```python
from build123d import *

# Parameters (mm, degrees)
F2_DEPTH = 10


with BuildPart() as f2:
    # F0 (on Front) → F2 (new body)
    with BuildSketch(Plane.XZ):
        with BuildLine():
            Line((0.211261, 25.041597), (0, 26.312215))
            ThreePointArc((0, 26.312215), (-0.220003, 26.826498), (-0.481302, 27.32108))
            ThreePointArc((-0.481302, 27.32108), (-0.825797, 27.312847), (-1.170161, 27.300274))
            ThreePointArc((-1.170161, 27.300274), (-1.401135, 26.790824), (-1.589699, 26.264201))
            Line((-1.589699, 26.264201), (-1.724216, 24.980969))
            Line((-1.724216, 24.980969), (-3.022362, 24.863022))
            Line((-3.022362, 24.863022), (-0.476655, 3.921135))
            ThreePointArc((-0.476655, 3.921135), (-0.222131, 3.943749), (0.033323, 3.949859))
            Line((0.033323, 3.949859), (0.211261, 25.041597))
        make_face()
    extrude(amount=F2_DEPTH)


with BuildPart() as f2_1:
    # F3: moved
    add(f2.part.moved(Location((0, 0, 0.5))))


solid = f2_1.part
```
Check sheet for the modelled part. Datum: model origin and axes. Units: mm. Coordinates: 2 decimals unless noted, no trailing zeros. Order: outer loops, then holes, each group sorted by start corner. A loop starts at its lowest first (then second) coordinate and runs counter-clockwise, first axis right, second up. Notation, with made-up numbers: (67, 25) -> (114, 25) arc R18 ccw to (114, 30) -> close; hole circle Ø2 at (-14.5, 48). An arc over 180 degrees is marked (long way). Write each question's results on one line, items separated by ' | '. Start each with the question number.
1) Draft check along Z on faces 1 (the face through (-1.767, -4.93, 15.039)), 2 (the face through (-1, 0, 19)), 3 (the face through (-1.398, -4.93, 27.298)). Enter one of: pulls with the +Z half, pulls with the -Z half, needs draft (parallel to the pull), parting line crosses it, or undercut.
2) Section check C-C (x = -0.7). Enter the section's corners in (y, z), and give its area (3 significant figures).
3) Section check A-A (y = -1). Enter the section's corners in (x, z), and give its area (3 significant figures).
4) Material ranges on line 1 along X through (y, z) = (-4.5, 18); line 2 along X through (y, z) = (-0.25, 10); line 3 along Z through (x, y) = (-0.1, -4.25), recorded low to high.
5) Depth check by flat-ended pin: pin 1 (1 mm diameter, centred on y = -4, z = 9.5, fed in from +X); pin 2 (2 mm diameter, centred on y = -3, z = 9.5, fed in from -X). Enter the tip coordinate at first touch or a pass-through.
6) Section check B-B (z = 15). Enter the section's corners in (x, y).
Checked values:
1) face 1: pulls with the -Z half | face 2: needs draft | face 3: pulls with the +Z half
2) outline: (-10, 6.26) -> (0, 6.26) -> (0, 27.82) -> (-10, 27.82) -> close | area: 216 mm²
3) outline: (-3.02, 25.36) -> (-0.48, 4.42) arc R3.95 cw to (0.03, 4.45) -> (0.21, 25.54) -> (0, 26.81) arc R6.84 ccw to (-0.48, 27.82) arc R27.35 ccw to (-1.17, 27.8) arc R6.84 ccw to (-1.59, 26.76) -> (-1.72, 25.48) -> close | area: 43.0 mm²
4) line 1: -2.13 to 0.15 | line 2: -1.15 to 0.08 | line 3: 4.45 to 27.06
5) pin 1: x = 0.08 | pin 2: x = -1.22
6) outline: (-1.76, -10) -> (0.12, -10) -> (0.12, 0) -> (-1.76, 0) -> close
